CAD build for the part. Positions are in the model's coordinates, mm. A direction names the side the tool comes from. Give positions to 0.01 mm unless a question says otherwise; leave off trailing zeros. Order: outer loops, then holes, each group sorted by start corner. A loop starts at its lowest first (then second) coordinate and runs counter-clockwise, first axis right, second up. Notation, with made-up numbers: (76.25, -10.5) -> (113.25, -10.5) arc R32 cw to (113.25, 24.5) -> close; hole circle Ø3 at (31, -4.75). An arc over 180 degrees is marked (long way). Use one line per item in the form item = value. Start each with the question number.
1) Tool access for faces 1 (the face through (1.23, 16.1, 78.94)), 2 (the face through (1, 89, 88)): list every direction of +Z, -Z, +X, -X, +Y, -Y with a clear straight run to the whole face (end or side of a thin tool).
2) Cut at C-C, the plane z = 63.5. Give the cut face in (x, y), and give its area (3 significant figures).
3) Cut at D-D, the plane y = 41. Give the cut face in (x, z).
4) Cut at B-B, the plane y = 65. Give the cut face in (x, z), and give its area (3 significant figures).
5) Drop flat-ended pins along their axis: P1, Ø4, axis at x = -3, z = 32, coming from the +Y side; P2, Ø6, axis at y = 15.25, z = 9.5, coming from the -X side; P3, Ø3, axis at x = -4, y = 31, coming from the -Z side; P4, Ø2, axis at x = 0, z = 74, coming from the -Y side. Give the stop position or say it passes through.
6) Cut at A-A, the plane z = 36.5. Give the cut face in (x, y), and give its area (4 significant figures).
7) Mould opens along Y. For faces 3 (the face through (-3, 25, 43)), 4 (the face through (1, 97, 37)), 5 (the face through (1.23, 72.97, 60.6)) say: pulls with the +Y half, pulls with the -Y half, needs draft (parallel to the pull), parting line crosses it, or undercut.
8) Probe line 1 (Y direction, x = 1.25, z = 9.5); line 2 (Z direction, x = 1.5, y = 65); line 3 (Y direction, x = -3, z = 42.8). List the from-to ranges inside material, lowest first.
from build123d import *

# Parameters (mm, degrees)
F2_DEPTH = 2.5
F1_R     = 1.8
F1_R_2   = 2
F1_R_3   = 3.5
F1_R_4   = 2.3
F1_R_5   = 1.6
F1_R_6   = 2.7
F1_R_7   = 1.85
F1_R_8   = 1.45
F3_DEPTH = 2.501
F4_W     = 8
F4_H     = 3
F5_DEPTH = 5.5
F6_R     = 1
F7_DEPTH = 45.001


with BuildPart() as f2:
    # F0 (on Right) → F2 (new body)
    with BuildSketch(Plane.YZ):
        with BuildLine():
            Line((0, 40.5), (0, 0))
            Line((0, 0), (97, 0))
            Line((97, 0), (97, 75.5))
            Line((97, 75.5), (81, 100.5))
            Line((81, 100.5), (62.435909, 100.5))
            ThreePointArc((62.435909, 100.5), (43.402845, 88.81449), (22.058582, 95.389522))
            Line((22.058582, 95.389522), (13.745146, 96.307334))
            Line((13.745146, 96.307334), (12, 96.5))
            ThreePointArc((12, 96.5), (4.082951, 89.649058), (9.725713, 80.830084))
            Line((9.725713, 80.830084), (22.650574, 76.997597))
            ThreePointArc((22.650574, 76.997597), (33.091215, 63.506399), (23.611014, 49.323833))
            Line((23.611014, 49.323833), (0, 40.5))
        make_face()
    extrude(amount=F2_DEPTH)

    # F1 (on Right) → F3 (cut, through all)
    with BuildSketch(Plane.YZ):
        with Locations((65, 98)):
            Circle(F1_R)
        with Locations((65, 70.5)):
            Circle(F1_R_2)
        with Locations((65, 63.5)):
            Circle(F1_R_3)
        with Locations((58.937822, 60)):
            Circle(F1_R_2)
        with Locations((71.062178, 60)):
            Circle(F1_R_2)
        with Locations((12, 88.5)):
            Circle(F1_R_4)
        with Locations((4, 36.5)):
            Circle(F1_R_5)
        with Locations((4, 29)):
            Circle(F1_R_6)
        with Locations((4, 21.5)):
            Circle(F1_R_5)
        with Locations((15.25, 9.5)):
            Circle(F1_R_7)
        with Locations((23.25, 9.5)):
            Circle(F1_R_8)
        with Locations((48.5, 9.5)):
            Circle(F1_R_7)
        with Locations((81.75, 9.5)):
            Circle(F1_R_7)
        with Locations((73.75, 9.5)):
            Circle(F1_R_8)
    extrude(amount=F3_DEPTH, mode=Mode.SUBTRACT)

    # F4 (on Right) → F5 (join)
    with BuildSketch(Plane.YZ):
        with Locations((29, 43.5)):
            Rectangle(F4_W, F4_H)
    extrude(amount=-F5_DEPTH)

    # F6 (on face) → F7 (cut, through all)
    with BuildSketch(Plane.XY.offset(45)):
        with Locations((-3, 27.5)):
            Circle(F6_R)
    extrude(amount=-F7_DEPTH, mode=Mode.SUBTRACT)


solid = f2.part
Result:
q1.face_1 = +X, -X, -Y
q1.face_2 = +Z, +X, -X, +Y
q2.outline = (0, 33.09) -> (2.5, 33.09) -> (2.5, 61.5) -> (0, 61.5) -> close; (0, 68.5) -> (2.5, 68.5) -> (2.5, 97) -> (0, 97) -> close
q2.area = 142 mm²
q3.outline = (0, 0) -> (2.5, 0) -> (2.5, 88.62) -> (0, 88.62) -> close
q4.outline = (0, 0) -> (2.5, 0) -> (2.5, 60) -> (0, 60) -> close; (0, 67) -> (2.5, 67) -> (2.5, 68.5) -> (0, 68.5) -> close; (0, 72.5) -> (2.5, 72.5) -> (2.5, 96.2) -> (0, 96.2) -> close; (0, 99.8) -> (2.5, 99.8) -> (2.5, 100.5) -> (0, 100.5) -> close
q4.area = 215 mm²
q5.P1 = through
q5.P2 = 0
q5.P3 = 42
q5.P4 = 26.82
q6.outline = (0, 0) -> (2.5, 0) -> (2.5, 2.4) -> (0, 2.4) -> close; (0, 5.6) -> (2.5, 5.6) -> (2.5, 97) -> (0, 97) -> close
q6.area = 234.5 mm²
q7.face_3 = pulls with the -Y half
q7.face_4 = pulls with the +Y half
q7.face_5 = undercut
q8.line_1 = 0 to 13.4, 17.1 to 21.8, 24.7 to 46.65, 50.35 to 72.3, 75.2 to 79.9, 83.6 to 97
q8.line_2 = 0 to 60, 67 to 68.5, 72.5 to 96.2, 99.8 to 100.5
q8.line_3 = 25 to 26.5, 28.5 to 33
